from build123d import *

# Parameters (mm, degrees)
SKETCH1_R           = 14.5
BOSS_EXTRUDE1_DEPTH = 1.5
SKETCH2_R           = 12.5
BOSS_EXTRUDE2_DEPTH = 20
SKETCH3_R           = 14.5
BOSS_EXTRUDE3_DEPTH = 1.5
SKETCH4_R           = 11
CUT_EXTRUDE1_DEPTH  = 6
SKETCH5_R           = 1.5
CUT_EXTRUDE2_DEPTH  = 17
SKETCH6_R           = 3
CUT_EXTRUDE3_DEPTH  = 1


with BuildPart() as part:
    # Sketch1 → Boss-Extrude1 (new body)
    with BuildSketch(Plane(origin=(0, 0, 0), x_dir=(0, 0, -1), z_dir=(1, 0, 0))):
        Circle(SKETCH1_R)
    extrude(amount=BOSS_EXTRUDE1_DEPTH)

    # Sketch2 → Boss-Extrude2 (add)
    with BuildSketch(Plane(origin=(1.5, 0, 0), x_dir=(0, 0, -1), z_dir=(1, 0, 0))):
        Circle(SKETCH2_R)
    extrude(amount=BOSS_EXTRUDE2_DEPTH)

    # Sketch3 → Boss-Extrude3 (add)
    with BuildSketch(Plane(origin=(21.5, 0, 0), x_dir=(0, 0, -1), z_dir=(1, 0, 0))):
        Circle(SKETCH3_R)
    extrude(amount=BOSS_EXTRUDE3_DEPTH)

    # Sketch4 → Cut-Extrude1 (cut)
    with BuildSketch(Plane(origin=(23, 0, 0), x_dir=(0, 0, -1), z_dir=(1, 0, 0))):
        Circle(SKETCH4_R)
    extrude(amount=-CUT_EXTRUDE1_DEPTH, mode=Mode.SUBTRACT)

    # Sketch5 → Cut-Extrude2 (cut)
    with BuildSketch(Plane(origin=(17, 0, 0), x_dir=(0, 0, -1), z_dir=(1, 0, 0))):
        with Locations((0, 8)):
            Circle(SKETCH5_R)
        with Locations((8, 0)):
            Circle(SKETCH5_R)
        with Locations((0, -8)):
            Circle(SKETCH5_R)
        with Locations((-8, 0)):
            Circle(SKETCH5_R)
    extrude(amount=-CUT_EXTRUDE2_DEPTH, mode=Mode.SUBTRACT)

    # Sketch6 → Cut-Extrude3 (cut)
    with BuildSketch(Plane(origin=(17, 0, 0), x_dir=(0, 0, -1), z_dir=(1, 0, 0))):
        with Locations((0, 8)):
            Circle(SKETCH6_R)
        with Locations((8, 0)):
            Circle(SKETCH6_R)
        with Locations((0, -8)):
            Circle(SKETCH6_R)
        with Locations((-8, 0)):
            Circle(SKETCH6_R)
    extrude(amount=-CUT_EXTRUDE3_DEPTH, mode=Mode.SUBTRACT)


solid = part.part
Could you check a few things on this model? Use its own coordinates, in mm. A direction names the side the tool comes from. Coordinates: 2 decimals unless noted, no trailing zeros. Loops run counter-clockwise (first coordinate to the right, second up) from the corner with the lowest first, then second, coordinate; pieces in that order, holes last. Notation, with made-up numbers: (44, 1) -> (80, 1) arc R11 ccw to (80, 15) -> close; hole circle Ø2 at (85.5, -9.5). An arc over 180 degrees is marked (long way). Answer in a Markdown table with one row per item.
(1) If I drill on probe 1 along Y at (x, z) = (11.5, 0); probe 2 along X at (y, z) = (12.5, -7.25); probe 3 along Y at (x, z) = (20.85, 0), over which ranges is the centre line in solid material (lowest first)?
Results found:
| item | result |
|---|---|
| probe 1 | y = -12.5 to -9.5, -6.5 to 6.5, 9.5 to 12.5 |
| probe 2 | x = 0 to 1.5, 21.5 to 23 |
| probe 3 | y = -12.5 to -11, 11 to 12.5 |
(2) Imagine slicing it at D-D (z = 0.75). Give the number of separate pieces and of enclosed holes in the cut face, plus the area to 3 significant figures.
Results found:
| item | result |
|---|---|
| separate pieces | 3 |
| enclosed holes | 0 |
| area | 360 mm^2 |
(3) Imagine slicing it at B-B (x = 13.75). List the corners of the cut face in (y, z) for me, plus the area to 3 significant figures.
Results found:
| item | result |
|---|---|
| outline | circle Ø25 at (0, 0); hole circle Ø3 at (-8, 0); hole circle Ø3 at (0, -8); hole circle Ø3 at (0, 8); hole circle Ø3 at (8, 0) |
| area | 463 mm^2 |
(4) Imagine slicing it at C-C (z = 8.5). List the corners of the cut face in (x, y) for me.
Results found:
| item | result |
|---|---|
| outline | (0, -11.75) -> (1.5, -11.75) -> (1.5, -9.17) -> (21.5, -9.17) -> (21.5, -11.75) -> (23, -11.75) -> (23, -6.98) -> (17, -6.98) -> (17, -2.96) -> (16, -2.96) -> (16, -1.41) -> (0, -1.41) -> close; (0, 1.41) -> (16, 1.41) -> (16, 2.96) -> (17, 2.96) -> (17, 6.98) -> (23, 6.98) -> (23, 11.75) -> (21.5, 11.75) -> (21.5, 9.17) -> (1.5, 9.17) -> (1.5, 11.75) -> (0, 11.75) -> close |
(5) Thinking about a two-plate mould opening in X: for faces 1 (the face through (16.51, -1.15, -10.77)), 2 (the face through (1.5, 7, 11)), 3 (the face through (0, 0, 0)), 4 (the face through (16, -9.3, -1.3)), which applies, released by +X, released by -X, zero draft, split by the parting line, or undercut?
Results found:
| item | result |
|---|---|
| face 1 | zero draft |
| face 2 | undercut |
| face 3 | released by -X |
| face 4 | released by +X |
(6) Will these pins go through, and if not, where does the flat tip stop? pin 1 Ø5 at (y, z) = (-8, -1.5) entering from +X; pin 2 Ø1.8 at (y, z) = (1, -7.5) entering from +X; pin 3 Ø12 at (x, y) = (10, 9) entering from -Z; pin 4 Ø1.8 at (y, z) = (0, -8) entering from +X.
Results found:
| item | result |
|---|---|
| pin 1 | stops at x = 17 |
| pin 2 | stops at x = 16 |
| pin 3 | stops at z = -12.13 |
| pin 4 | passes through |
(7) For faces 5 (the face through (16.51, -1.15, 5.23)), 6 (the face through (21.5, 7, 11)), 7 (the face through (22.24, -12.864, -6.691)), which set-ups out of +Z, -Z, +X, -X, +Y, -Y let a thin tool reach every point of the face, with its end or its side?
Results found:
| item | result |
|---|---|
| face 5 | +X |
| face 6 | none |
| face 7 | +X, -X |
(8) Imagine slicing it at A-A (y = 8). List the corners of the cut face in (x, z) for me.
Results found:
| item | result |
|---|---|
| outline | (0, -12.09) -> (1.5, -12.09) -> (1.5, -9.6) -> (21.5, -9.6) -> (21.5, -12.09) -> (23, -12.09) -> (23, -7.55) -> (17, -7.55) -> (17, -3) -> (16, -3) -> (16, -1.5) -> (0, -1.5) -> close; (0, 1.5) -> (16, 1.5) -> (16, 3) -> (17, 3) -> (17, 7.55) -> (23, 7.55) -> (23, 12.09) -> (21.5, 12.09) -> (21.5, 9.6) -> (1.5, 9.6) -> (1.5, 12.09) -> (0, 12.09) -> close |
